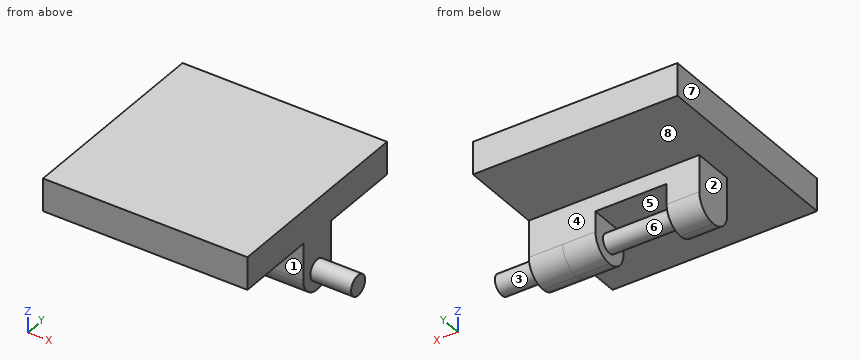
```python
from build123d import *

# Parameters (mm, degrees)
SKETCH1_R            = 12.7
BOSS_EXTRUDE3_DEPTH  = 152.4
SKETCH9_R            = 6.35
BOSS_EXTRUDE6_DEPTH  = 19.05
SKETCH16_W           = 25.4
SKETCH16_H           = 63.5
CUT_EXTRUDE2_DEPTH   = 155.762931731
SKETCH17_W           = 25.4
SKETCH17_H           = 63.5
CUT_EXTRUDE3_DEPTH   = 155.762931731
SKETCH19_R           = 2.54
CUT_EXTRUDE5_DEPTH   = 155.762931731
SKETCH21_W           = 21.59
SKETCH21_H           = 12.7
BOSS_EXTRUDE8_DEPTH  = 12.7
BOSS_EXTRUDE9_DEPTH  = 6.35
SKETCH25_R           = 3.175
CUT_EXTRUDE7_DEPTH   = 21.59
SKETCH29_R           = 2.921
BOSS_EXTRUDE10_DEPTH = 35.814
FILLET2_R            = 6.35
FILLET3_R            = 6.35
SKETCH31_W           = 63.5
SKETCH31_H           = 63.5
BOSS_EXTRUDE11_DEPTH = 10.16
SKETCH32_W           = 127
SKETCH32_H           = 307.417558359
CUT_EXTRUDE8_DEPTH   = 195.047688304
SKETCH33_W           = 21.59
SKETCH33_H           = 12.7
CUT_EXTRUDE9_DEPTH   = 195.047688304
SKETCH29_2_R         = 2.921
BOSS_EXTRUDE12_DEPTH = 35.814
SKETCH37_W           = 17.78
SKETCH37_H           = 12.7
BOSS_EXTRUDE13_DEPTH = 10.541
FILLET5_R            = 6.35
SKETCH38_R           = 3.175
BOSS_EXTRUDE14_DEPTH = 12.7


with BuildPart() as part:
    # Sketch1 → Boss-Extrude3 (new, symmetric)
    with BuildSketch(Plane.XY):
        with Locations(Location((0, 0, 0), (0, 0, 180))):
            Circle(SKETCH1_R)
    extrude(amount=BOSS_EXTRUDE3_DEPTH, both=True)

    # Sketch9 → Boss-Extrude6 (add, symmetric)
    with BuildSketch(Plane(origin=(0, 0, 0), x_dir=(0, 0, -1), z_dir=(1, 0, 0))):
        with Locations((-25.4, 0)):
            Circle(SKETCH9_R)
    extrude(amount=BOSS_EXTRUDE6_DEPTH, both=True)

    # Sketch16 → Cut-Extrude2 (cut, through all)
    with BuildSketch(Plane(origin=(0, -6.35, 0), x_dir=(1, 0, 0), z_dir=(0, 1, 0))):
        with Locations((0, 120.65)):
            Rectangle(SKETCH16_W, SKETCH16_H)
    extrude(amount=-CUT_EXTRUDE2_DEPTH, mode=Mode.SUBTRACT)

    # Sketch17 → Cut-Extrude3 (cut, through all)
    with BuildSketch(Plane(origin=(0, 6.35, 0), x_dir=(1, 0, 0), z_dir=(0, 1, 0))):
        with Locations((0, 120.65)):
            Rectangle(SKETCH17_W, SKETCH17_H)
    extrude(amount=CUT_EXTRUDE3_DEPTH, mode=Mode.SUBTRACT)

    # Sketch19 → Cut-Extrude5 (cut, through all)
    with BuildSketch(Plane(origin=(0, 6.35, 0), x_dir=(1, 0, 0), z_dir=(0, 1, 0))):
        with Locations(Location((0, 100.80625, 0), (0, 0, 270))):
            Circle(SKETCH19_R)
        with Locations(Location((0, 136.525, 0), (0, 0, 270))):
            Circle(SKETCH19_R)
    extrude(amount=-CUT_EXTRUDE5_DEPTH, mode=Mode.SUBTRACT)

    # Sketch21 → Boss-Extrude8 (add)
    with BuildSketch(Plane.XY.offset(152.4)):
        Rectangle(SKETCH21_W, SKETCH21_H)
    extrude(amount=BOSS_EXTRUDE8_DEPTH)

    # Sketch25 → Cut-Extrude7 (cut)
    with BuildSketch(Plane.ZY.offset(10.795)):
        with Locations(Location((158.75, 0, 0), (0, 0, 270))):
            Circle(SKETCH25_R)
    extrude(amount=-CUT_EXTRUDE7_DEPTH, mode=Mode.SUBTRACT)

    # Fillet3
    fillet3_edges = [part.edges().sort_by_distance(p)[0] for p in [
        (0, -6.35, 165.1),
        (0, 6.35, 165.1),
    ]]
    fillet(fillet3_edges, radius=FILLET3_R - 0.0001)  # a hair under: the kernel refuses the full size

    # Sketch32 → Cut-Extrude8 (cut, through all)
    with BuildSketch(Plane(origin=(0, 31.75, 0), x_dir=(1, 0, 0), z_dir=(0, 1, 0))):
        with Locations((19.549323816, 1.30877918)):
            Rectangle(SKETCH32_W, SKETCH32_H)
    extrude(amount=-CUT_EXTRUDE8_DEPTH, mode=Mode.SUBTRACT)


with BuildPart() as body_2:
    # Sketch27 → Boss-Extrude9 (new, symmetric)
    with BuildSketch(Plane(origin=(0, 0, 0), x_dir=(1, 0, 0), z_dir=(0, 1, 0))):
        Polygon((0, -165.354), (11.049, -165.354), (11.049, -152.654), (21.209, -152.654), (21.209, -170.434), (-21.209, -170.434), (-21.209, -152.654), (-11.049, -152.654), (-11.049, -165.354), align=None)
    extrude(amount=BOSS_EXTRUDE9_DEPTH, both=True)

    # Sketch29 → Boss-Extrude10 (add)
    with BuildSketch(Plane.ZY.offset(21.209)):
        with Locations((158.827896988, 0)):
            Circle(SKETCH29_R)
    extrude(amount=-BOSS_EXTRUDE10_DEPTH)

    # Fillet2
    fillet2_edges = [body_2.edges().sort_by_distance(p)[0] for p in [
        (16.129, -6.35, 152.654),
        (16.129, 6.35, 152.654),
        (-16.129, -6.35, 152.654),
        (-16.129, 6.35, 152.654),
    ]]
    fillet(fillet2_edges, radius=FILLET2_R - 0.0001)  # a hair under: the kernel refuses the full size

    # Sketch31 → Boss-Extrude11 (add)
    with BuildSketch(Plane.XY.offset(170.434)):
        Rectangle(SKETCH31_W, SKETCH31_H)
    extrude(amount=BOSS_EXTRUDE11_DEPTH)


with BuildPart() as cut_extrude9_tool:
    # Sketch33 → Cut-Extrude9 (new, through all)
    with BuildSketch(Plane(origin=(0, 31.75, 0), x_dir=(1, 0, 0), z_dir=(0, 1, 0))):
        with Locations((0, -158.75)):
            Rectangle(SKETCH33_W, SKETCH33_H)
    extrude(amount=-CUT_EXTRUDE9_DEPTH)


with BuildPart() as part_1:
    add(part.part)

    # Cut-Extrude9: cut by cut_extrude9_tool
    add(cut_extrude9_tool.part, mode=Mode.SUBTRACT)


with BuildPart() as body_2_1:
    add(body_2.part)

    # Cut-Extrude9: cut by cut_extrude9_tool
    add(cut_extrude9_tool.part, mode=Mode.SUBTRACT)

    # Sketch29<2> → Boss-Extrude12 (add)
    with BuildSketch(Plane.ZY.offset(21.209)):
        with Locations((158.827896988, 0)):
            Circle(SKETCH29_2_R)
    extrude(amount=-BOSS_EXTRUDE12_DEPTH)

    # Sketch37 → Boss-Extrude13 (add)
    with BuildSketch(Plane(origin=(21.209, 0, 0), x_dir=(0, 0, -1), z_dir=(1, 0, 0))):
        with Locations((-161.544, 0)):
            Rectangle(SKETCH37_W, SKETCH37_H)
    extrude(amount=BOSS_EXTRUDE13_DEPTH)

    # Fillet5
    fillet5_edges = [body_2_1.edges().sort_by_distance(p)[0] for p in [
        (26.4795, -6.35, 152.654),
        (26.4795, 6.35, 152.654),
    ]]
    fillet(fillet5_edges, radius=FILLET5_R - 0.0001)  # a hair under: the kernel refuses the full size

    # Sketch38 → Boss-Extrude14 (add)
    with BuildSketch(Plane(origin=(31.75, 0, 0), x_dir=(0, 0, -1), z_dir=(1, 0, 0))):
        with Locations(Location((-158.827896988, 0, 0), (0, 0, 180))):
            Circle(SKETCH38_R)
    extrude(amount=BOSS_EXTRUDE14_DEPTH)


solid = body_2_1.part
```
Verification items for the finished model (mm, model axes). Face numbers are marked on the shaded views. A direction names the side the tool comes from. Coordinates: 2 decimals unless noted, no trailing zeros. Loops run counter-clockwise (first coordinate to the right, second up) from the corner with the lowest first, then second, coordinate; pieces in that order, holes last. Notation, with made-up numbers: (-29.5, -24.5) -> (8.5, -24.5) arc R27 cw to (8.5, 13.5) -> close; hole circle Ø3 at (-10.75, 30). An arc over 180 degrees is marked (long way). Answer in a Markdown table with one row per item. Add a question column.
1. Section check D-D, the plane z = 166.5. Enter the section's corners in (x, y).
2. Draft check along X on the marked faces 6, 7 and 8. Enter one of: +X half, -X half, draft (parallel to the pull), parting line (faces both ways), or undercut.
3. Access from +Z, -Z, +X, -X, +Y, -Y to the whole of each face (thin tool, end or side, straight path). Record for the marked faces 1, 2, 3, 4 and 5.
4. Section check A-A, the plane x = 0. Enter the section's corners in (y, z), then the cut area to 3 significant figures.
5. Material ranges on probe 1 along Y at (x, z) = (-8, 167.5); probe 2 along X at (y, z) = (-2, 173.75); probe 3 along Z at (x, y) = (-15, -9.5), recorded low to high. Write a range as [from, to].
6. Depth check by flat-ended pin: P1, Ø1.5, axis at x = -3, z = 159, coming from the -Y side; P2, Ø1, axis at y = -23.5, z = 175, coming from the +X side; P3, Ø5, axis at y = -3, z = 155, coming from the -X side. Enter the tip coordinate at first touch or a pass-through.
7. Section check C-C, the plane y = 15. Enter the section's corners in (x, z).
Derived:
| question | item | result |
|---|---|---|
| 1 | outline | (-21.21, -6.35) -> (31.75, -6.35) -> (31.75, 6.35) -> (-21.21, 6.35) -> close |
| 2 | face 6 | undercut |
| 2 | face 7 | -X half |
| 2 | face 8 | draft |
| 3 | face 1 | -Z, +X, -X, -Y |
| 3 | face 2 | -Z, -X, +Y, -Y |
| 3 | face 3 | +X |
| 3 | face 4 | -Z, +X, -X, +Y |
| 3 | face 5 | +Y, -Y |
| 4 | outline | (-31.75, 170.43) -> (-6.35, 170.43) -> (-6.35, 165.35) -> (6.35, 165.35) -> (6.35, 170.43) -> (31.75, 170.43) -> (31.75, 180.59) -> (-31.75, 180.59) -> close; circle Ø5.84 at (0, 158.83) |
| 4 | area | 736 mm² |
| 5 | probe 1 | y = [-6.35, 6.35] |
| 5 | probe 2 | x = [-31.75, 31.75] |
| 5 | probe 3 | z = [170.43, 180.59] |
| 6 | P1 | stops at y = -2.92 |
| 6 | P2 | stops at x = 31.75 |
| 6 | P3 | stops at x = -21.21 |
| 7 | outline | (-31.75, 170.43) -> (31.75, 170.43) -> (31.75, 180.59) -> (-31.75, 180.59) -> close |
